The figure shows three views and two pictorial views of one solid part (mm, origin at its lowest corner). Answer the questions. Give positions to 0.01 mm unless a question says otherwise; leave off trailing zeros. Order: outer loops, then holes, each group sorted by start corner. A loop starts at its lowest first (then second) coordinate and runs counter-clockwise, first axis right, second up. Notation, with made-up numbers: (21, 89) - (73, 89) arc R18 ccw to (73, 102) - close; hole circle Ø3 at (-23, 45.5). An arc over 180 degrees is marked (long way). Answer as CSV lines item,"result". Start each with the question number.
1. Consider line 1 along Y through (x, z) = (1.4, 85.09); line 2 along Y through (x, z) = (0.9, 152.4); line 3 along Z through (x, y) = (1, 76). Determine where each line is inside the solid, lowest interval first. Write a range as [from, to].
2. Section B-B on z = 17.78 is taken. Give the vertices of the cut face in (x, y), and give its area (3 significant figures).
3. Section A-A on x = 0.65 is taken. Give the vertices of the cut face in (y, z), and give its area (3 significant figures).
4. Flat-ended cylindrical pins translate along their axes: pin 1 (1.5 mm diameter, centred on y = 34.5, z = 67.5, fed in from -X); pin 2 (1 mm diameter, centred on x = 1, y = 146, fed in from -Z); pin 3 (0.8 mm diameter, centred on x = 1.5, z = 79.5, fed in from -Y); pin 4 (1 mm diameter, centred on x = 1, z = 54, fed in from +Y). Find the tip coordinate at first contact, or state that the pin passes through.
5. Section D-D on z = 85.09 is taken. Give the vertices of the cut face in (x, y), and give its area (3 significant figures).
6. Section C-C on y = 81.5 is taken. Give the vertices of the cut face in (x, z).
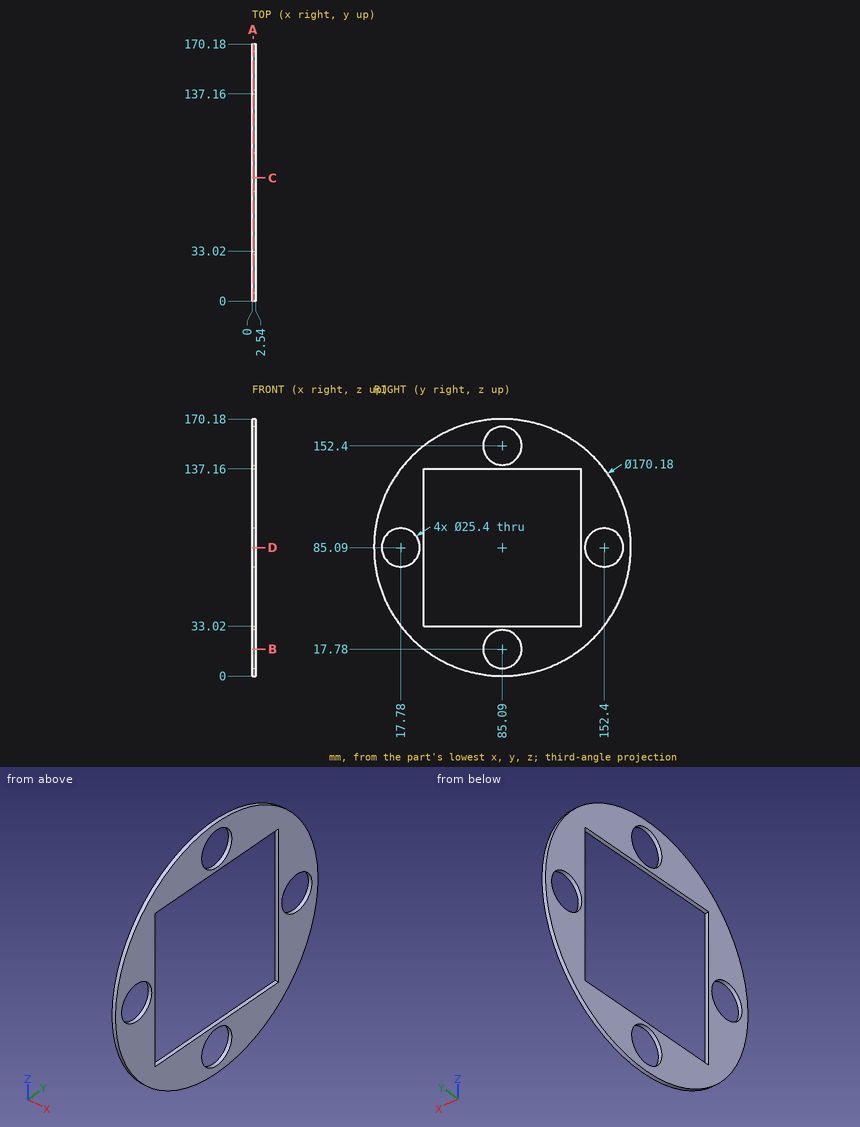
Checks:
1,line 1,"y = [0, 5.08], [30.48, 33.02], [137.16, 139.7], [165.1, 170.18]"
1,line 2,"y = [33.04, 72.39], [97.79, 137.14]"
1,line 3,"z = [0.49, 8.91], [26.65, 33.02], [137.16, 143.53], [161.27, 169.69]"
2,outline,"(0, 33.04) - (2.54, 33.04) - (2.54, 72.39) - (0, 72.39) - close; (0, 97.79) - (2.54, 97.79) - (2.54, 137.14) - (0, 137.14) - close"
2,area,"200 mm²"
3,outline,"circle Ø170.18 at (85.09, 85.09); hole circle Ø25.4 at (17.78, 85.09); hole (33.02, 33.02) - (137.16, 33.02) - (137.16, 137.16) - (33.02, 137.16) - close; hole circle Ø25.4 at (85.09, 17.78); hole circle Ø25.4 at (85.09, 152.4); hole circle Ø25.4 at (152.4, 85.09)"
3,area,"9,870 mm²"
4,pin 1,"passes through"
4,pin 2,"stops at z = 25.17"
4,pin 3,"stops at y = 0.16"
4,pin 4,"stops at y = 164.49"
5,outline,"(0, 0) - (2.54, 0) - (2.54, 5.08) - (0, 5.08) - close; (0, 30.48) - (2.54, 30.48) - (2.54, 33.02) - (0, 33.02) - close; (0, 137.16) - (2.54, 137.16) - (2.54, 139.7) - (0, 139.7) - close; (0, 165.1) - (2.54, 165.1) - (2.54, 170.18) - (0, 170.18) - close"
5,area,"38.7 mm²"
6,outline,"(0, 0.08) - (2.54, 0.08) - (2.54, 5.6) - (0, 5.6) - close; (0, 29.96) - (2.54, 29.96) - (2.54, 33.02) - (0, 33.02) - close; (0, 137.16) - (2.54, 137.16) - (2.54, 140.22) - (0, 140.22) - close; (0, 164.58) - (2.54, 164.58) - (2.54, 170.1) - (0, 170.1) - close"
